Build history of the part. All positions in model axes, mm. A direction names the side the tool comes from. Round coordinates to 2 decimals unless told otherwise and drop trailing zeros. Write each loop counter-clockwise with the first axis right and the second up, starting at its lowest first coordinate (ties: lowest second). Pieces come first, ordered by that corner, then holes.
Item 1: Band-saw the part on C-C, the plane z = 452.5. Write the cut outline in (x, y).
Item 2: Band-saw the part on B-B, the plane y = -163. Write the cut outline in (x, z).
Item 3: Band-saw the part on D-D, the plane x = 0. Count the separate pieces of the cut face and the enclosed holes in it, then the cut area to 3 significant figures.
Item 4: Drop flat-ended pins along their axis: pin 1 Ø1 at (x, z) = (53.5, -419) entering from -Y; pin 2 Ø20 at (x, z) = (-14, -361) entering from -Y. Give the stop position or say it passes through.
Item 5: 3-axis set-ups, long thin cutter, end or side, ignore diameter. For faces 1 (the cylindrical face through (68.97, -9.86, 640.58)), 2 (the flat face through (2, -170, 761.394)), 3 (the cylindrical face through (-21.551, -280.146, -356.874)): which of +Z, -Z, +X, -X, +Y, -Y reach the whole face in a straight line?
Item 6: Band-saw the part on A-A, the plane x = -134.5. Write the cut outline in (y, z), then the cut area to 3 significant figures.
Item 7: Wall check: probe 1 along Z at (x, y) = (-40.5, -168); probe 2 along Z at (x, y) = (-138, -180.5); probe 3 along X at (y, z) = (-181, 641). Give the ranges that are in metal, low to high.
Item 8: Mould opens along X. For faces 4 (the flat face through (-160, -324, 3)), 5 (the cylindrical face through (59.835, -9.86, -287.067)) say: +X half, -X half, draft (parallel to the pull), parting line (faces both ways), or undercut.
```python
from build123d import *

# Parameters (mm, degrees)
F0_W     = 340
F0_H     = 1560
F0_R     = 120
F1_DEPTH = 20
F2_W     = 304
F2_H     = 18
F3_DEPTH = 304
F4_DEPTH = 286
F5_R     = 120
F6_DEPTH = 18
F8_DEPTH = 18
F7_R     = 120
F9_DEPTH = 18


with BuildPart() as f1:
    # F0 (on Front) → F1 (new body)
    with BuildSketch(Plane.XZ):
        with Locations((4.462467, -0.60629)):
            Rectangle(F0_W, F0_H)
        with Locations((4.462467, -540.60629)):
            Circle(F0_R, mode=Mode.SUBTRACT)
        with Locations((4.462467, -180.60629)):
            Circle(F0_R, mode=Mode.SUBTRACT)
        with Locations((4.462467, 179.39371)):
            Circle(F0_R, mode=Mode.SUBTRACT)
        with Locations((4.462467, 539.39371)):
            Circle(F0_R, mode=Mode.SUBTRACT)
    extrude(amount=F1_DEPTH)

    # F2 (on face) → F3 (join)
    with BuildSketch(Plane.XZ.offset(20)):
        Polygon((-165.537533, 779.39371), (-165.537533, -780.60629), (-147.537533, -780.60629), (-147.537533, -762.60629), (-147.537533, -366), (-147.537533, -348), (-147.537533, -18), (-147.537533, 0), (-147.537533, 18), (-147.537533, 348), (-147.537533, 366), (-147.537533, 761.39371), (-147.537533, 779.39371), align=None)
        with Locations((4.462467, 770.39371)):
            Rectangle(F2_W, F2_H)
        Polygon((156.462467, -762.60629), (156.462467, -780.60629), (174.462467, -780.60629), (174.462467, 779.39371), (156.462467, 779.39371), (156.462467, 761.39371), (156.462467, 366), (156.462467, 348), (156.462467, 18), (156.462467, 0), (156.462467, -18), (156.462467, -348), (156.462467, -366), align=None)
        with Locations((4.462467, -771.60629)):
            Rectangle(F2_W, F2_H)
    extrude(amount=F3_DEPTH)

    # F2 (on face) → F4 (join)
    with BuildSketch(Plane.XZ.offset(20)):
        with Locations((4.462467, -357)):
            Rectangle(F2_W, F2_H)
        with Locations((4.462467, 9)):
            Rectangle(F2_W, F2_H)
        with Locations((4.462467, -9)):
            Rectangle(F2_W, F2_H)
        with Locations((4.462467, 357)):
            Rectangle(F2_W, F2_H)
    extrude(amount=F4_DEPTH)

    # F5 (on face) → F6 (cut)
    with BuildSketch(Plane.XY.offset(366)):
        with Locations((0, -163)):
            Circle(F5_R)
    extrude(amount=-F6_DEPTH, mode=Mode.SUBTRACT)

    # F5 (on face) → F8 (cut)
    with BuildSketch(Plane.XY.offset(366)):
        with Locations((0, -163)):
            Circle(F5_R)
    extrude(amount=-F8_DEPTH, mode=Mode.SUBTRACT)

    # F7 (on face) → F9 (cut)
    with BuildSketch(Plane.XY.offset(-348)):
        with Locations((4.462467, -163)):
            Circle(F7_R)
    extrude(amount=-F9_DEPTH, mode=Mode.SUBTRACT)


solid = f1.part
```
Results:
1. outline: (-165.54, -324) - (-147.54, -324) - (-147.54, -20) - (-78.3, -20) - (-78.3, 0) - (-165.54, 0) - close; (87.22, -20) - (156.46, -20) - (156.46, -324) - (174.46, -324) - (174.46, 0) - (87.22, 0) - close
2. outline: (-165.54, -780.61) - (174.46, -780.61) - (174.46, 779.39) - (-165.54, 779.39) - close; hole (-147.54, -762.61) - (156.46, -762.61) - (156.46, -366) - (124.46, -366) - (124.46, -348) - (156.46, -348) - (156.46, -18) - (-147.54, -18) - (-147.54, -348) - (-115.54, -348) - (-115.54, -366) - (-147.54, -366) - close; hole (-147.54, 18) - (156.46, 18) - (156.46, 348) - (120, 348) - (120, 366) - (156.46, 366) - (156.46, 761.39) - (-147.54, 761.39) - (-147.54, 366) - (-120, 366) - (-120, 348) - (-147.54, 348) - close
3. separate pieces: 7
3. enclosed holes: 0
3. area: 34,900 mm2
4. pin 1: stops at y = -20
4. pin 2: stops at y = -306
5. face 1: +Y, -Y
5. face 2: -Y
5. face 3: none
6. outline: (-324, -780.61) - (0, -780.61) - (0, 779.39) - (-324, 779.39) - (-324, 761.39) - (-20, 761.39) - (-20, 366) - (-306, 366) - (-306, 348) - (-20, 348) - (-20, 18) - (-306, 18) - (-306, -18) - (-20, -18) - (-20, -348) - (-306, -348) - (-306, -366) - (-20, -366) - (-20, -762.61) - (-324, -762.61) - close
6. area: 62,700 mm2
7. probe 1: z = -780.61 to -762.61, -18 to 18, 761.39 to 779.39
7. probe 2: z = -780.61 to -762.61, -366 to -348, -18 to 18, 348 to 366, 761.39 to 779.39
7. probe 3: x = -165.54 to -147.54, 156.46 to 174.46
8. face 4: draft
8. face 5: undercut
